```python
from build123d import *

# Parameters (mm, degrees)
BOSS_EXTRUDE1_DEPTH = 69
CUT_EXTRUDE1_DEPTH  = 20.3
CHAMFER1_SIZE       = 0.5


with BuildPart() as part:
    # Sketch1 → Boss-Extrude1 (new body)
    with BuildSketch(Plane(origin=(0, 0, 0), x_dir=(1, 0, 0), z_dir=(0, 1, 0))):
        with BuildLine():
            ThreePointArc((2.625, 0), (-1.215138881, 2.326813809), (-1.5, -2.154210992))
            Line((-1.5, -2.154210992), (1.5, -2.154210992))
            ThreePointArc((1.5, -2.154210992), (2.326813809, -1.215138881), (2.625, 0))
        make_face()
        with BuildLine():
            Line((1.5, -2.154210992), (-1.5, -2.154210992))
            ThreePointArc((-1.5, -2.154210992), (0, -2.625), (1.5, -2.154210992))
        make_face()
    extrude(amount=BOSS_EXTRUDE1_DEPTH)

    # Sketch1<3> → Cut-Extrude1 (cut)
    with BuildSketch(Plane(origin=(0, 0, 0), x_dir=(1, 0, 0), z_dir=(0, 1, 0))):
        with BuildLine():
            Line((1.5, -2.154210992), (-1.5, -2.154210992))
            ThreePointArc((-1.5, -2.154210992), (0, -2.625), (1.5, -2.154210992))
        make_face()
    extrude(amount=CUT_EXTRUDE1_DEPTH, mode=Mode.SUBTRACT)

    # Chamfer1
    # the kernel refuses this chamfer: 0.5 mm, written as the material it takes off along each edge
    with BuildSketch(Plane(origin=(2.785841494, 0, 2.154210992), x_dir=(0, 0.9996219169112968, 0.027495876610586494), z_dir=(-1, 0, 0))) as chamfer1_piece_1:
        Polygon((CHAMFER1_SIZE * 0.999621916911, CHAMFER1_SIZE * 0.0274958766106), (-CHAMFER1_SIZE * 0.0274958766106, CHAMFER1_SIZE * 0.999621916911), (0, 0), align=None)
    extrude(amount=5.571682988, mode=Mode.SUBTRACT)
    with BuildSketch(Plane(origin=(0, 0, 0), x_dir=(0.11608616482785569, 0, 0.9932391465984212), z_dir=(-0.9932391465984212, 0, 0.11608616482785569))) as chamfer1_piece_2:
        Polygon((2.625, CHAMFER1_SIZE), (2.625 - CHAMFER1_SIZE, 0), (2.625, 0), align=None)
    revolve(axis=Axis((0, 0, 0), (0, 1, 0)), revolution_arc=346.667445344, mode=Mode.SUBTRACT)


solid = part.part
```
For this review, take the finished solid that the model builds, in its own axes (mm). A direction names the side the tool comes from. Give positions to 0.01 mm unless a question says otherwise; leave off trailing zeros. Write each loop counter-clockwise with the first axis right and the second up, starting at its lowest first coordinate (ties: lowest second). Pieces come first, ordered by that corner, then holes. Notation, with made-up numbers: M 74.5,3.5 L 133.5,3.5 A23 ccw 133.5,29.5 Z; hole C -37,40.5 d8. An arc over 180 degrees is marked long. One line per item, written item: value.
1) Take a section at B-B, the plane y = 7. Write out the cut boundary in (x, z) (3 decimals).
Results are:
outline: M -1.5,2.154 A2.625 ccw long 1.5,2.154 Z
2) Take a section at A-A, the plane x = 0. Write out the cut boundary in (y, z) (3 decimals), then the cut area to 3 significant figures.
Results are:
outline: M 0,-2.125 L 0.5,-2.625 L 69,-2.625 L 69,2.625 L 20.3,2.625 L 20.3,2.154 L 0.5,2.154 L 0,1.654 Z
area: 352 mm²
3) For line 1 (Z direction, x = 0.15, y = 27.5); line 2 (Z direction, x = 0.05, y = 6), list the stretches that pass through material, from the lowest coordinate up. Write a range as from..to.
Results are:
line 1: z = -2.62..2.62
line 2: z = -2.62..2.15
4) Take a section at C-C, the plane y = 42.5. Write out the cut boundary in (x, z) (3 decimals).
Results are:
outline: C 0,0 d5.25
5) For P1, Ø2, axis at x = -1.5, y = 60, coming from the -Z side, flat-tipped, find the tip position at first contact; note if it passes through.
Results are:
P1: stops at z = -2.58
6) For faces 1 (the flat face through (0, 69, 0)), 2 (the flat face through (0, 10, 2.154)), list the 3-axis set-ups (+Z, -Z, +X, -X, +Y, -Y) from which the entire face can be reached by the end or side of a thin tool; tool diameter is ignored.
Results are:
face 1: +Z, -Z, +X, -X, +Y
face 2: +Z, +X, -X, -Y
